For this review, use the dimensioned drawing (mm, ordinates from the lowest corner) and the shaded views. Give positions to 0.01 mm unless a question says otherwise; leave off trailing zeros. Write each loop counter-clockwise with the first axis right and the second up, starting at its lowest first coordinate (ties: lowest second). Pieces come first, ordered by that corner, then holes.
1) We need section D-D on z = 34.5. Give the boundary of the cut face in (x, y), and give its area (3 significant figures).
2) We need section A-A on x = 120. Give the boundary of the cut face in (y, z), and give its area (3 significant figures).
3) Wall thickness on line 1 along Y through (x, z) = (120, 47); line 2 along X through (y, z) = (121.5, 21.5); line 3 along Z through (x, y) = (15, 102): over which ranges is each line inside the solid? List them lowest first.
4) We need section C-C on z = 66. Give the boundary of the cut face in (x, y).
5) Draft analysis for pull direction Y (two halves, no side actions). For the marked faces 1, 2 and 3, state which applies: pulls with the +Y half, pulls with the -Y half, needs draft (parallel to the pull), parting line crosses it, or undercut.
6) For P1, Ø5, axis at x = 167.5, z = 25, coming from the -Y side; P2, Ø2, axis at y = 140.5, z = 38, coming from the -X side; P3, Ø6, axis at x = 186.5, z = 25.5, coming from the -Y side, all flat-tipped, find the tip position at first contact; note any pin that passes through.
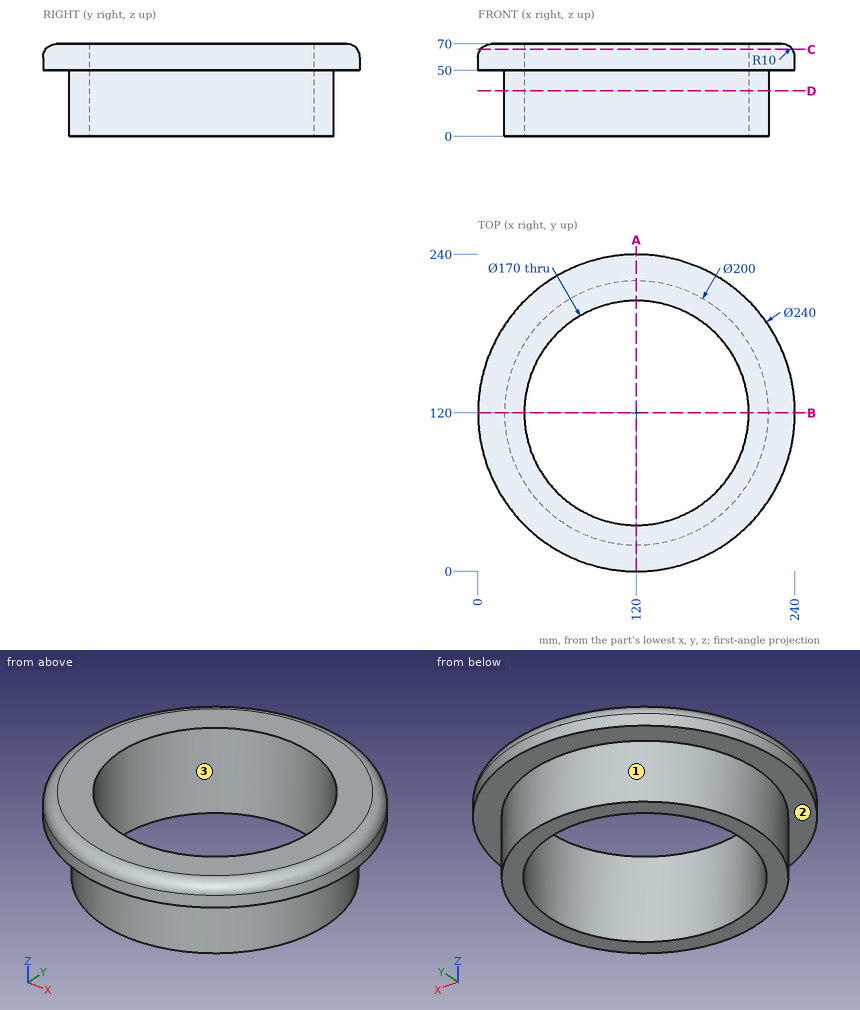
Results list:
1. outline: circle Ø200 at (120, 120); hole circle Ø170 at (120, 120)
1. area: 8,720 mm2
2. outline: (0, 50) - (20, 50) - (20, 0) - (35, 0) - (35, 70) - (10, 70) arc R10 ccw to (0, 60) - close; (205, 0) - (220, 0) - (220, 50) - (240, 50) - (240, 60) arc R10 ccw to (230, 70) - (205, 70) - close
2. area: 2,860 mm2
3. line 1: y = 20 to 35, 205 to 220
3. line 2: x = 20.01 to 35.01, 204.99 to 219.99
3. line 3: z = 50 to 70
4. outline: circle Ø236 at (120, 120); hole circle Ø170 at (120, 120)
5. face 1: parting line crosses it
5. face 2: needs draft
5. face 3: undercut
6. P1: stops at y = 30.7
6. P2: stops at x = 21.92
6. P3: stops at y = 42.75
